For this review, use the dimensioned drawing (mm, ordinates from the lowest corner) and the shaded views. A direction names the side the tool comes from. Coordinates: 2 decimals unless noted, no trailing zeros. Order: outer loops, then holes, each group sorted by start corner. A loop starts at its lowest first (then second) coordinate and runs counter-clockwise, first axis right, second up. Notation, with made-up numbers: M 63.5,61 L 82.5,61 A11 cw 82.5,79 Z; hole C 86,32.5 d1. An arc over 180 degrees is marked long. Answer in a Markdown table with one row per item.
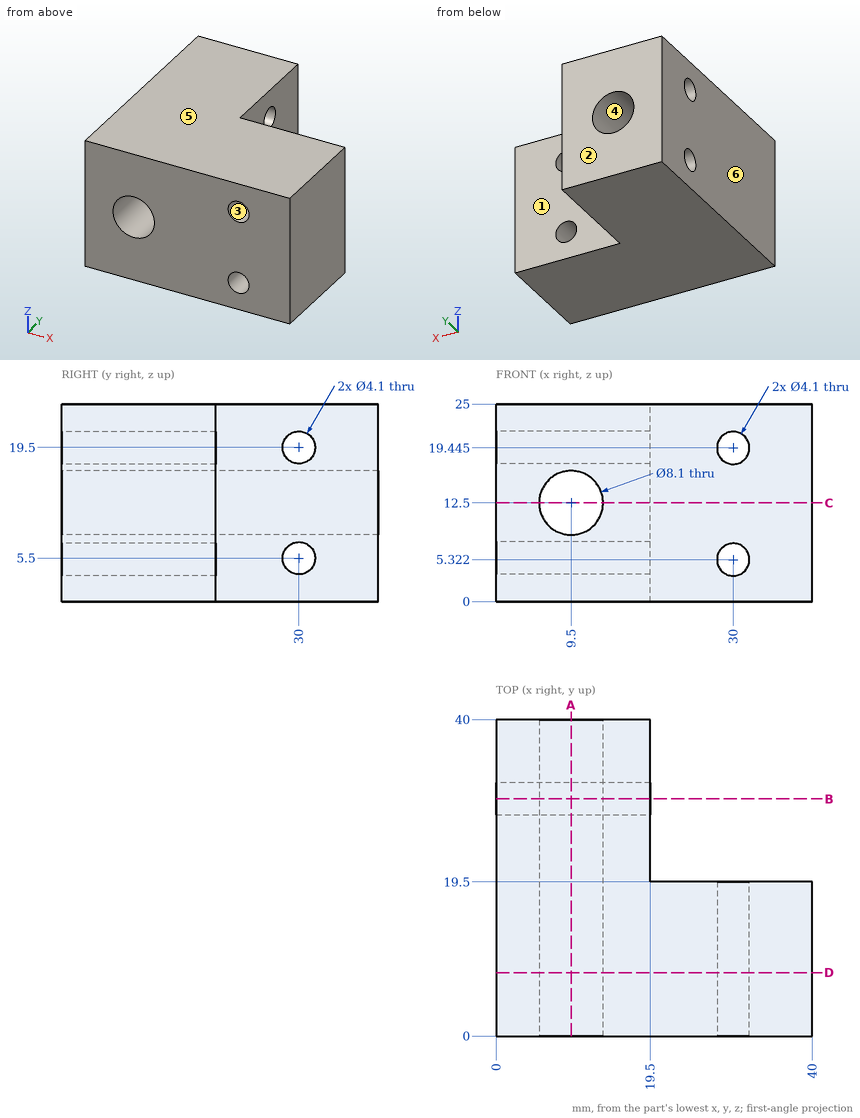
(1) Add section D-D, the plane y = 8. Give the boundary of the cut face in (x, z) (3 decimals), and give its area (3 significant figures).
Return value:
| item | result |
|---|---|
| outline | M 0,0 L 40,0 L 40,25 L 0,25 Z; hole C 9.5,12.5 d8.1; hole C 30,5.322 d4.1; hole C 30,19.445 d4.1 |
| area | 922 mm2 |
(2) Add section B-B, the plane y = 30. Give the boundary of the cut face in (x, z).
Return value:
| item | result |
|---|---|
| outline | M 0,0 L 19.5,0 L 19.5,3.45 L 0,3.45 Z; M 0,7.55 L 19.5,7.55 L 19.5,17.45 L 0,17.45 Z; M 0,21.55 L 19.5,21.55 L 19.5,25 L 0,25 Z; hole C 9.5,12.5 d8.1 |
(3) Draft analysis for pull direction Z (two halves, no side actions). For the marked faces 3, 4, 5 and 6, state which applies: pulls with the +Z half, pulls with the -Z half, needs draft (parallel to the pull), parting line crosses it, or undercut.
Return value:
| item | result |
|---|---|
| face 3 | undercut |
| face 4 | undercut |
| face 5 | pulls with the +Z half |
| face 6 | needs draft |
(4) Insertion check: pin 1 Ø6 at (y, z) = (30, 3) entering from +X; pin 2 Ø6 at (x, z) = (25.5, 7) entering from +Y; pin 3 Ø3.5 at (x, z) = (30, 19.45) entering from -Y. Each pin has a flat end and moves straight along its axis. Give the tip position at first contact, or say it passes through.
Return value:
| item | result |
|---|---|
| pin 1 | stops at x = 19.5 |
| pin 2 | stops at y = 19.5 |
| pin 3 | passes through |
(5) For the marked faces 1 and 2, list the 3-axis set-ups (+Z, -Z, +X, -X, +Y, -Y) from which the entire face can be reached by the end or side of a thin tool; tool diameter is ignored.
Return value:
| item | result |
|---|---|
| face 1 | +Z, -Z, +X, +Y |
| face 2 | +Z, -Z, +X, -X, +Y |
(6) For line 1 along Z through (x, y) = (5, 30); line 2 along Z through (x, y) = (30, 14) (3 decimals); line 3 along Z through (x, y) = (9.5, 17), list the stretches that pass through material, from the lowest coordinate up. Write a range as from..to.
Return value:
| item | result |
|---|---|
| line 1 | z = 0..3.45, 7.55..17.45, 21.55..25 |
| line 2 | z = 0..3.272, 7.372..17.395, 21.495..25 |
| line 3 | z = 0..8.45, 16.55..25 |
(7) Add section A-A, the plane x = 9.5. Give the boundary of the cut face in (y, z).
Return value:
| item | result |
|---|---|
| outline | M 0,0 L 40,0 L 40,8.45 L 0,8.45 Z; M 0,16.55 L 40,16.55 L 40,25 L 0,25 Z; hole C 30,5.5 d4.1; hole C 30,19.5 d4.1 |
(8) Add section C-C, the plane z = 12.5. Give the boundary of the cut face in (x, y).
Return value:
| item | result |
|---|---|
| outline | M 0,0 L 5.45,0 L 5.45,40 L 0,40 Z; M 13.55,0 L 40,0 L 40,19.5 L 19.5,19.5 L 19.5,40 L 13.55,40 Z |
